```python
from build123d import *

# Parameters (mm, degrees)
SKETCH1_R           = 127
BOSS_EXTRUDE1_DEPTH = 19.05
CUT_EXTRUDE1_DEPTH  = 19.05
BOSS_EXTRUDE2_DEPTH = 43.18
FILLET1_R           = 3.81
CUT_EXTRUDE4_START  = -5.08
SKETCH7_R           = 36.385525633
SKETCH7_R_2         = 34.07613751
CUT_EXTRUDE4_DEPTH  = 2.54
CUT_EXTRUDE5_START  = -36.83
SKETCH8_R           = 36.385525633
SKETCH8_R_2         = 34.07613751
CUT_EXTRUDE5_DEPTH  = 2.54
SKETCH4_R           = 152.4
SKETCH4_R_2         = 127
BOSS_EXTRUDE3_DEPTH = 190.5
CUT_EXTRUDE2_START  = 12.7
CUT_EXTRUDE2_DEPTH  = 12.7
CUT_EXTRUDE6_START  = -12.7
SKETCH6_R           = 3.51155
CUT_EXTRUDE6_DEPTH  = 171.45
BOSS_EXTRUDE4_DEPTH = 88.9
CUT_EXTRUDE8_DEPTH  = 88.9
FILLET2_R           = 1.016
CUT_EXTRUDE9_START  = -16.51
CUT_EXTRUDE9_DEPTH  = 16.51
CUT_EXTRUDE12_START = -171.45
SKETCH14_R          = 152.4
SKETCH14_R_2        = 127
CUT_EXTRUDE12_DEPTH = 171.45
SKETCH15_R          = 152.4
CUT_EXTRUDE13_DEPTH = 6.35
SKETCH17_W          = 19.05
SKETCH17_H          = 41.16468875
CUT_EXTRUDE15_DEPTH = 88.9
CHAMFER2_SIZE       = 12.7


with BuildPart() as part:
    # Sketch1 → Boss-Extrude1 (new body)
    with BuildSketch(Plane(origin=(0, 0, 0), x_dir=(1, 0, 0), z_dir=(0, 1, 0))):
        with Locations(Location((0, 0, 0), (0, 0, 90))):
            Circle(SKETCH1_R)
    extrude(amount=BOSS_EXTRUDE1_DEPTH)

    # Sketch2 → Cut-Extrude1 (cut)
    with BuildSketch(Plane(origin=(0, 19.05, 0), x_dir=(1, 0, 0), z_dir=(0, 1, 0))):
        with BuildLine():
            Line((-16.764, 16.002), (-16.764, -16.002))
            Line((-16.764, -16.002), (0.678310948, -15.224897184))
            ThreePointArc((0.678310948, -15.224897184), (15.24, 0), (0.678310948, 15.224897184))
            Line((0.678310948, 15.224897184), (-16.764, 16.002))
        make_face()
    extrude(amount=-CUT_EXTRUDE1_DEPTH, mode=Mode.SUBTRACT)

    # Sketch3 → Boss-Extrude2 (add)
    with BuildSketch(Plane(origin=(-38.1, 0, 0), x_dir=(0, 0, -1), z_dir=(1, 0, 0))):
        with BuildLine():
            Line((-25.4, 19.05), (25.4, 19.05))
            Line((25.4, 19.05), (25.4, 48.26))
            ThreePointArc((25.4, 48.26), (0, 22.86), (-25.4, 48.26))
            Line((-25.4, 48.26), (-25.4, 19.05))
        make_face()
    extrude(amount=-BOSS_EXTRUDE2_DEPTH)

    # Fillet1
    fillet1_edges = [part.edges().sort_by_distance(p)[0] for p in [
        (-59.69, 48.26, 25.4),
        (-59.69, 48.26, -25.4),
    ]]
    fillet(fillet1_edges, radius=FILLET1_R - 0.0001)  # a hair under: the kernel refuses the full size

    # Sketch7 → Cut-Extrude4 (cut, symmetric)
    with BuildSketch(Plane(origin=(-38.1, 0, 0), x_dir=(0, 0, -1), z_dir=(1, 0, 0)).offset(CUT_EXTRUDE4_START)):
        with Locations((0, 48.26)):
            Circle(SKETCH7_R)
        with Locations((0, 48.26)):
            Circle(SKETCH7_R_2, mode=Mode.SUBTRACT)
    extrude(amount=CUT_EXTRUDE4_DEPTH, both=True, mode=Mode.SUBTRACT)

    # Sketch8 → Cut-Extrude5 (cut, symmetric)
    with BuildSketch(Plane(origin=(-38.1, 0, -38.1), x_dir=(0, 0, -1), z_dir=(1, 0, 0)).offset(CUT_EXTRUDE5_START)):
        with Locations((-38.1, 48.26)):
            Circle(SKETCH8_R)
        with Locations((-38.1, 48.26)):
            Circle(SKETCH8_R_2, mode=Mode.SUBTRACT)
    extrude(amount=CUT_EXTRUDE5_DEPTH, both=True, mode=Mode.SUBTRACT)

    # Sketch4 → Boss-Extrude3 (add)
    with BuildSketch(Plane(origin=(0, 0, 0), x_dir=(1, 0, 0), z_dir=(0, 1, 0))):
        with Locations(Location((0, 0, 0), (0, 0, 270))):
            Circle(SKETCH4_R)
        with Locations(Location((0, 0, 0), (0, 0, 270))):
            Circle(SKETCH4_R_2, mode=Mode.SUBTRACT)
    extrude(amount=BOSS_EXTRUDE3_DEPTH)

    # Sketch5 → Cut-Extrude2 (cut)
    with BuildSketch(Plane(origin=(0, 190.5, -228.6), x_dir=(1, 0, 0), z_dir=(0, -1, 0)).offset(CUT_EXTRUDE2_START)):
        with BuildLine():
            Line((-25.4, 351.737617729), (-25.4, 378.868426491))
            ThreePointArc((-25.4, 378.868426491), (0, 381), (25.4, 378.868426491))
            Line((25.4, 378.868426491), (25.4, 351.737617729))
            ThreePointArc((25.4, 351.737617729), (62.865, 337.485374018), (93.940305115, 312.165854121))
            Line((93.940305115, 312.165854121), (117.436274728, 325.731258501))
            ThreePointArc((117.436274728, 325.731258501), (131.982271537, 304.8), (142.836274728, 281.737167989))
            Line((142.836274728, 281.737167989), (119.340305115, 268.171763608))
            ThreePointArc((119.340305115, 268.171763608), (125.73, 228.6), (119.340305115, 189.028236392))
            Line((119.340305115, 189.028236392), (142.836274728, 175.462832011))
            ThreePointArc((142.836274728, 175.462832011), (131.982271537, 152.4), (117.436274728, 131.468741499))
            Line((117.436274728, 131.468741499), (93.940305115, 145.034145879))
            ThreePointArc((93.940305115, 145.034145879), (62.865, 119.714625982), (25.4, 105.462382271))
            Line((25.4, 105.462382271), (25.4, 78.331573509))
            ThreePointArc((25.4, 78.331573509), (0, 76.2), (-25.4, 78.331573509))
            Line((-25.4, 78.331573509), (-25.4, 105.462382271))
            ThreePointArc((-25.4, 105.462382271), (-62.865, 119.714625982), (-93.940305115, 145.034145879))
            Line((-93.940305115, 145.034145879), (-117.436274728, 131.468741499))
            ThreePointArc((-117.436274728, 131.468741499), (-131.982271537, 152.4), (-142.836274728, 175.462832011))
            Line((-142.836274728, 175.462832011), (-119.340305115, 189.028236392))
            ThreePointArc((-119.340305115, 189.028236392), (-125.73, 228.6), (-119.340305115, 268.171763608))
            Line((-119.340305115, 268.171763608), (-142.836274728, 281.737167989))
            ThreePointArc((-142.836274728, 281.737167989), (-131.982271537, 304.8), (-117.436274728, 325.731258501))
            Line((-117.436274728, 325.731258501), (-93.940305115, 312.165854121))
            ThreePointArc((-93.940305115, 312.165854121), (-62.865, 337.485374018), (-25.4, 351.737617729))
        make_face()
    extrude(amount=-CUT_EXTRUDE2_DEPTH, mode=Mode.SUBTRACT)

    # Sketch6 → Cut-Extrude6 (cut)
    with BuildSketch(Plane(origin=(0, 190.5, 0), x_dir=(1, 0, 0), z_dir=(0, 1, 0)).offset(CUT_EXTRUDE6_START)):
        with Locations(Location((0, 139.7, 0), (0, 0, 90))):
            Circle(SKETCH6_R)
        with Locations(Location((120.983748909, 69.85, 0), (0, 0, 90))):
            Circle(SKETCH6_R)
        with Locations(Location((120.983748909, -69.85, 0), (0, 0, 90))):
            Circle(SKETCH6_R)
        with Locations(Location((0, -139.7, 0), (0, 0, 90))):
            Circle(SKETCH6_R)
        with Locations(Location((-120.983748909, -69.85, 0), (0, 0, 90))):
            Circle(SKETCH6_R)
        with Locations(Location((-120.983748909, 69.85, 0), (0, 0, 90))):
            Circle(SKETCH6_R)
    extrude(amount=-CUT_EXTRUDE6_DEPTH, mode=Mode.SUBTRACT)

    # Sketch9 → Boss-Extrude4 (add)
    with BuildSketch(Plane(origin=(0, 19.05, 0), x_dir=(1, 0, 0), z_dir=(0, 1, 0))):
        with BuildLine():
            Line((38.1, 121.15027858), (38.1, -121.15027858))
            ThreePointArc((38.1, -121.15027858), (47.781803057, -117.668599451), (57.15, -113.414626482))
            Line((57.15, -113.414626482), (57.15, 113.414626482))
            ThreePointArc((57.15, 113.414626482), (47.781803057, 117.668599451), (38.1, 121.15027858))
        make_face()
    extrude(amount=BOSS_EXTRUDE4_DEPTH)

    # Sketch10 → Cut-Extrude8 (cut)
    with BuildSketch(Plane(origin=(0, 107.95, 0), x_dir=(1, 0, 0), z_dir=(0, 1, 0))):
        Polygon((57.15, -50.8), (57.15, 50.8), (44.45, 65.935270626), (44.45, -65.935270626), align=None)
    extrude(amount=-CUT_EXTRUDE8_DEPTH, mode=Mode.SUBTRACT)

    # Fillet2
    fillet2_edges = [part.edges().sort_by_distance(p)[0] for p in [
        (44.45, 63.5, 65.935270626),
        (44.45, 63.5, -65.935270626),
        (57.15, 63.5, -50.8),
        (57.15, 63.5, 50.8),
    ]]
    fillet(fillet2_edges, radius=FILLET2_R)

    # Sketch11 → Cut-Extrude9 (cut)
    with BuildSketch(Plane.XZ.offset(CUT_EXTRUDE9_START)):
        with BuildLine():
            Line((-29.464, 29.280418015), (-29.464, -29.280418015))
            Line((-29.464, -29.280418015), (1.243570072, -27.912311504))
            ThreePointArc((1.243570072, -27.912311504), (27.94, 0), (1.243570072, 27.912311504))
            Line((1.243570072, 27.912311504), (-29.464, 29.280418015))
        make_face()
        with BuildLine():
            Line((-16.764, 16.002), (-16.764, -16.002))
            Line((-16.764, -16.002), (0.678310948, -15.224897184))
            ThreePointArc((0.678310948, -15.224897184), (15.24, 0), (0.678310948, 15.224897184))
            Line((0.678310948, 15.224897184), (-16.764, 16.002))
        make_face(mode=Mode.SUBTRACT)
    extrude(amount=CUT_EXTRUDE9_DEPTH, mode=Mode.SUBTRACT)

    # Sketch14 → Cut-Extrude12 (cut)
    with BuildSketch(Plane(origin=(0, 190.5, 0), x_dir=(1, 0, 0), z_dir=(0, 1, 0)).offset(CUT_EXTRUDE12_START)):
        with Locations(Location((0, 0, 0), (0, 0, 270))):
            Circle(SKETCH14_R)
        Circle(SKETCH14_R_2, mode=Mode.SUBTRACT)
    extrude(amount=CUT_EXTRUDE12_DEPTH, mode=Mode.SUBTRACT)

    # Sketch15 → Cut-Extrude13 (cut)
    with BuildSketch(Plane.XZ):
        with Locations(Location((0, 0, 0), (0, 0, 270))):
            Circle(SKETCH15_R)
    extrude(amount=-CUT_EXTRUDE13_DEPTH, mode=Mode.SUBTRACT)

    # Sketch17 → Cut-Extrude15 (cut)
    with BuildSketch(Plane(origin=(0, 107.95, 0), x_dir=(1, 0, 0), z_dir=(0, 1, 0))):
        with Locations((47.625, 100.567934205)):
            Rectangle(SKETCH17_W, SKETCH17_H)
        with Locations((47.625, -100.567934205)):
            Rectangle(SKETCH17_W, SKETCH17_H)
    extrude(amount=-CUT_EXTRUDE15_DEPTH, mode=Mode.SUBTRACT)

    # Chamfer2
    chamfer2_edges = [part.edges().sort_by_distance(p)[0] for p in [
        (38.1, 19.05, 0),
        (47.625, 19.05, -79.98558983),
        (47.625, 19.05, 79.98558983),
    ]]
    chamfer(chamfer2_edges, length=CHAMFER2_SIZE)


solid = part.part
```
Work out the finished part from the listing and answer in its coordinate system (mm). A direction names the side the tool comes from. Give positions to 0.01 mm unless a question says otherwise; leave off trailing zeros. Write each loop counter-clockwise with the first axis right and the second up, starting at its lowest first coordinate (ties: lowest second). Pieces come first, ordered by that corner, then holes. Notation, with made-up numbers: (77.25, -5.75) -> (86.25, -5.75) arc R32 ccw to (86.25, 33.25) -> close; hole circle Ø10 at (52.5, 87.25). An arc over 180 degrees is marked (long way). Write each question's results on one line, items separated by ' | '.
1. Find section C-C on x = 85. Determine the outline of the cut face in (y, z), and give its area (3 significant figures).
Data:
outline: (6.35, -126.49) -> (19.05, -126.49) -> (19.05, 126.49) -> (6.35, 126.49) -> close | area: 3,210 mm^2
2. Straight lines are drawn through the part: L1, parallel to Z at x = -3, y = 17.5; L2, parallel to Y at x = 89, z = 95.5; L3, parallel to X at y = 76, z = 18. For each, find the intervals that lie inside material, in ascending order.
Data:
L1: -152.37 to -141.53, -137.87 to -15.39, 15.39 to 137.87, 141.53 to 152.37 | L2: 6.35 to 19.05 | L3: 38.1 to 44.45
3. Each of these flat-tipped pins is pushed along its axis until it touches: pin 1 Ø14.5 at (y, z) = (29, 7.5) entering from +X; pin 2 Ø21 at (x, y) = (49.5, 84) entering from +Z; pin 3 Ø8 at (x, z) = (50, -96.5) entering from +Y; pin 4 Ø5.5 at (x, z) = (0, 139.7) entering from +Y. Where does it stop, or does it pass through?
Data:
pin 1: x = 44.45 | pin 2: z = 79.99 | pin 3: y = 19.24 | pin 4: through
4. Find section B-B on y = 101. Determine the outline of the cut face in (x, z).
Data:
outline: (38.1, -79.99) -> (57.15, -79.99) -> (57.15, -53.59) arc R1.02 ccw to (55.36, -52.94) -> (46.24, -63.8) arc R1.02 cw to (44.45, -63.14) -> (44.45, 63.14) arc R1.02 cw to (46.24, 63.8) -> (55.36, 52.94) arc R1.02 ccw to (57.15, 53.59) -> (57.15, 79.99) -> (38.1, 79.99) -> close
5. Find section A-A on z = 2.5. Give the number of separate pieces and of enclosed holes in the cut face, and give its area (3 significant figures).
Data:
separate pieces: 2 | enclosed holes: 2 | area: 4,000 mm^2
6. A tool of negligible diameter and unlimited length cuts with its end or side. For faces 4 (the flat face through (-59, 24, -25.4)), 5 (the flat face through (47, 70, 79.986)), 6 (the flat face through (31.66, 25.31, -1.3)), 7 (the flat face through (-20, 16.51, 0)), from which of +Z, -Z, +X, -X, +Y, -Y can it reach the whole face along a straight path? Write none if from no direction.
Data:
face 4: -Z, -X, +Y | face 5: +Z, +X, -X, +Y | face 6: +Z, -Z, +Y | face 7: -Y
7. Determine the mould class of faces 1 (the flat face through (57.15, 63, 69)), 2 (the flat face through (-29.464, 12, 0)), 3 (the flat face through (44.581, 25.311, 86.424)) for opening direction X: +X half, -X half, draft (parallel to the pull), parting line (faces both ways), or undercut.
Data:
face 1: +X half | face 2: undercut | face 3: draft
